```python
from build123d import *

# Parameters (mm, degrees)
SKETCH_W      = 50
SKETCH_H      = 35
PAD_DEPTH     = 10
SKETCH001_R   = 2
SKETCH001_R_2 = 2.5
SKETCH001_R_3 = 5
SKETCH001_W   = 4
SKETCH001_H   = 4
SKETCH001_W_2 = 6
SKETCH001_H_2 = 6
SKETCH001_W_3 = 10
SKETCH001_H_3 = 10
POCKET_DEPTH  = 10.001


with BuildPart() as part:
    # Sketch → Pad (new body)
    with BuildSketch(Plane.XY):
        Rectangle(SKETCH_W, SKETCH_H)
    extrude(amount=PAD_DEPTH)

    # Sketch001 (on Face6 of Pad) → Pocket (cut, through all)
    with BuildSketch(Plane.XY.offset(10)):
        with Locations((-15, 7.5)):
            Circle(SKETCH001_R)
        with Locations((0, 7.5)):
            Circle(SKETCH001_R_2)
        with Locations((15, 7.5)):
            Circle(SKETCH001_R_3)
        with Locations((-15, -7.5)):
            Rectangle(SKETCH001_W, SKETCH001_H)
        with Locations((0, -7.5)):
            Rectangle(SKETCH001_W_2, SKETCH001_H_2)
        with Locations((15, -7.5)):
            Rectangle(SKETCH001_W_3, SKETCH001_H_3)
    extrude(amount=-POCKET_DEPTH, mode=Mode.SUBTRACT)


solid = part.part
```
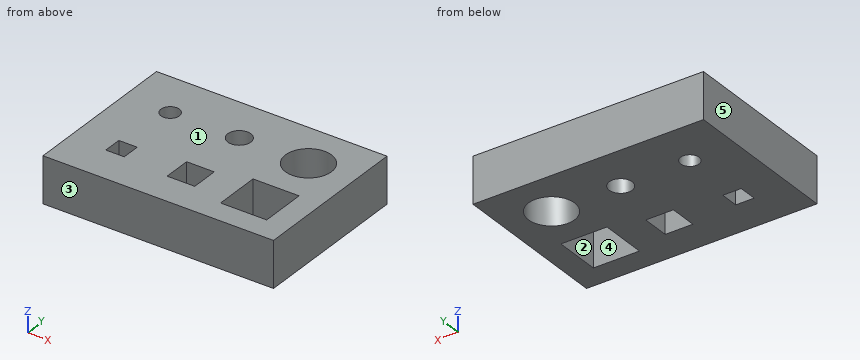
Here's how the part is built. I have some questions about the finished solid (model axes, mm). Face numbers are marked on the shaded views. A direction names the side the tool comes from. Round coordinates to 2 decimals unless told otherwise and drop trailing zeros. Loops run counter-clockwise (first coordinate to the right, second up) from the corner with the lowest first, then second, coordinate; pieces in that order, holes last. Notation, with made-up numbers: (9.25, 71) -> (21.25, 71) arc R11 cw to (21.25, 86) -> close; hole circle Ø6 at (88.25, 24.5). An arc over 180 degrees is marked (long way). Answer as CSV lines item,"result". Start each with the question number.
1. If we mould it in two halves opening along Y, with no side actions, what happens to the marked faces 1, 2 and 3? For each: pulls with the +Y half, pulls with the -Y half, needs draft (parallel to the pull), parting line crosses it, or undercut.
2. Imagine slicing it at D-D on y = -6.5. Write out the boundary of the cut face in (x, z), plus the area to 3 significant figures.
3. Imagine slicing it at B-B on y = 7.5. Write out the boundary of the cut face in (x, z).
4. Imagine slicing it at A-A on x = 15. Write out the boundary of the cut face in (y, z), plus the area to 3 significant figures.
5. I'm going to push flat-ended pins straight in: P1, Ø6, axis at x = 0, y = 7.5, coming from the -Z side; P2, Ø8, axis at x = 15, y = 7.5, coming from the -Z side. Where does each tip first touch, or does it pass through?
6. I need wall thicknesses on probe 1 along Y at (x, z) = (0, 6); probe 2 along Y at (x, z) = (15, 7.25); probe 3 along X at (y, z) = (-10, 8.25). Which ranges of each line are inside material? Lowest first, please. Write a range as from..to.
7. For the marked faces 4 and 5, which set-ups out of +Z, -Z, +X, -X, +Y, -Y let a thin tool reach every point of the face, with its end or its side?
8. Imagine slicing it at C-C on z = 5.75. Write out the boundary of the cut face in (x, y).
Solution:
1,face 1,"needs draft"
1,face 2,"undercut"
1,face 3,"pulls with the -Y half"
2,outline,"(-25, 0) -> (-17, 0) -> (-17, 10) -> (-25, 10) -> close; (-13, 0) -> (-3, 0) -> (-3, 10) -> (-13, 10) -> close; (3, 0) -> (10, 0) -> (10, 10) -> (3, 10) -> close; (20, 0) -> (25, 0) -> (25, 10) -> (20, 10) -> close"
2,area,"300 mm²"
3,outline,"(-25, 0) -> (-17, 0) -> (-17, 10) -> (-25, 10) -> close; (-13, 0) -> (-2.5, 0) -> (-2.5, 10) -> (-13, 10) -> close; (2.5, 0) -> (10, 0) -> (10, 10) -> (2.5, 10) -> close; (20, 0) -> (25, 0) -> (25, 10) -> (20, 10) -> close"
4,outline,"(-17.5, 0) -> (-12.5, 0) -> (-12.5, 10) -> (-17.5, 10) -> close; (-2.5, 0) -> (2.5, 0) -> (2.5, 10) -> (-2.5, 10) -> close; (12.5, 0) -> (17.5, 0) -> (17.5, 10) -> (12.5, 10) -> close"
4,area,"150 mm²"
5,P1,"z = 0"
5,P2,"through"
6,probe 1,"-17.5..-10.5, -4.5..5, 10..17.5"
6,probe 2,"-17.5..-12.5, -2.5..2.5, 12.5..17.5"
6,probe 3,"-25..-3, 3..10, 20..25"
7,face 4,"+Z, -Z"
7,face 5,"+Z, -Z, -X, +Y, -Y"
8,outline,"(-25, -17.5) -> (25, -17.5) -> (25, 17.5) -> (-25, 17.5) -> close; hole (-17, -9.5) -> (-13, -9.5) -> (-13, -5.5) -> (-17, -5.5) -> close; hole circle Ø4 at (-15, 7.5); hole (-3, -10.5) -> (3, -10.5) -> (3, -4.5) -> (-3, -4.5) -> close; hole circle Ø5 at (0, 7.5); hole (10, -12.5) -> (20, -12.5) -> (20, -2.5) -> (10, -2.5) -> close; hole circle Ø10 at (15, 7.5)"
